```python
from build123d import *

# Parameters (mm, degrees)
F0_W     = 32
F0_H     = 72
F1_DEPTH = 10
F3_D     = 6.6
F5_D     = 12
F6_SIZE  = 5


with BuildPart() as f1:
    # F0 (on Right) → F1 (new body)
    with BuildSketch(Plane.YZ):
        with Locations((16, 36)):
            Rectangle(F0_W, F0_H)
    extrude(amount=F1_DEPTH)

    # F3 (through all)
    with Locations(Plane.YZ.offset(10)):
        with Locations((10, 35), (10, 10)):
            Hole(F3_D / 2)

    # F5 (through all)
    with Locations(Plane.YZ.offset(10)):
        with Locations((20, 60)):
            Hole(F5_D / 2)

    # F6
    f6_edges = [f1.edges().sort_by_distance(p)[0] for p in [
        (5, 0, 72),
        (5, 32, 72),
    ]]
    chamfer(f6_edges, length=F6_SIZE)


solid = f1.part
```
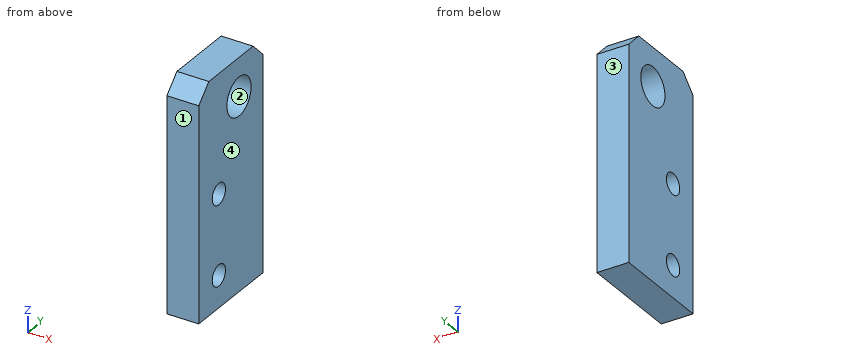
The listing builds one solid part. Answer for the finished solid, in the listing's coordinates (mm). Face numbers are marked on the shaded views. Round coordinates to 2 decimals unless told otherwise and drop trailing zeros. Loops run counter-clockwise (first coordinate to the right, second up) from the corner with the lowest first, then second, coordinate; pieces in that order, holes last. Notation, with made-up numbers: (47, -4) -> (81, -4) arc R23 ccw to (81, 9) -> close; hole circle Ø10 at (63.5, -19). An arc over 180 degrees is marked (long way). Use one line per item in the form item = value.
1. The part is cut by section A-A on y = 20. Determine the outline of the cut face in (x, z), and give its area (3 significant figures).
Answer key:
outline = (0, 0) -> (10, 0) -> (10, 54) -> (0, 54) -> close; (0, 66) -> (10, 66) -> (10, 72) -> (0, 72) -> close
area = 600 mm²
2. The part is cut by section C-C on y = 10. Determine the outline of the cut face in (x, z), and give its area (3 significant figures).
Answer key:
outline = (0, 0) -> (10, 0) -> (10, 6.7) -> (0, 6.7) -> close; (0, 13.3) -> (10, 13.3) -> (10, 31.7) -> (0, 31.7) -> close; (0, 38.3) -> (10, 38.3) -> (10, 72) -> (0, 72) -> close
area = 588 mm²
3. The part is cut by section B-B on z = 60. Determine the outline of the cut face in (x, y).
Answer key:
outline = (0, 0) -> (10, 0) -> (10, 14) -> (0, 14) -> close; (0, 26) -> (10, 26) -> (10, 32) -> (0, 32) -> close
4. The part is cut by section D-D on x = 6.25. Determine the outline of the cut face in (y, z), and give its area (3 significant figures).
Answer key:
outline = (0, 0) -> (32, 0) -> (32, 67) -> (27, 72) -> (5, 72) -> (0, 67) -> close; hole circle Ø6.6 at (10, 10); hole circle Ø6.6 at (10, 35); hole circle Ø12 at (20, 60)
area = 2,100 mm²
5. For a pull along Y with two mould halves and no side action, classify the marked faces 1, 2, 3 and 4 as released by +Y, released by -Y, zero draft, split by the parting line, or undercut.
Answer key:
face_1 = released by -Y
face_2 = undercut
face_3 = released by +Y
face_4 = zero draft
6. Find the intervals of material crossed by probe 1 along Z at (x, y) = (5.5, 10); probe 2 along Z at (x, y) = (6, 20); probe 3 along Z at (x, y) = (7.75, 8.5), in increasing order. Write a range as [from, to].
Answer key:
probe_1 = [0, 6.7], [13.3, 31.7], [38.3, 72]
probe_2 = [0, 54], [66, 72]
probe_3 = [0, 7.06], [12.94, 32.06], [37.94, 72]
